from build123d import *

# Parameters (mm, degrees)
ESQUISSE1_R             = 8
ESQUISSE1_R_2           = 1.6
BOSS_EXTRU_1_DEPTH      = 4
ESQUISSE3_R             = 1.6
ENL_V_MAT_EXTRU_1_DEPTH = 10
ENL_V_MAT_EXTRU_2_DEPTH = 5
ESQUISSE5_R             = 1.6
ENL_V_MAT_EXTRU_4_DEPTH = 5
ESQUISSE6_R             = 1.6
ESQUISSE6_R_2           = 1.621897971
ENL_V_MAT_EXTRU_5_DEPTH = 5
ENL_V_MAT_EXTRU_6_DEPTH = 5


with BuildPart() as part:
    # Esquisse1 → Boss.-Extru.1 (new body)
    with BuildSketch(Plane(origin=(0, 0, 0), x_dir=(1, 0, 0), z_dir=(0, 1, 0))):
        Polygon((-150, 0), (-150, 260), (-110, 300), (110, 300), (150, 260), (150, 0), align=None)
        with Locations(Location((-119.984856992, 30, 0), (0, 0, 270))):
            Circle(ESQUISSE1_R, mode=Mode.SUBTRACT)
        with Locations(Location((-120, 268, 0), (0, 0, 270))):
            Circle(ESQUISSE1_R, mode=Mode.SUBTRACT)
        with Locations(Location((120, 269.55960862, 0), (0, 0, 270))):
            Circle(ESQUISSE1_R, mode=Mode.SUBTRACT)
        with Locations(Location((-111.514718626, 276.485281374, 0), (0, 0, 270))):
            Circle(ESQUISSE1_R_2, mode=Mode.SUBTRACT)
        with Locations(Location((-128.485281374, 259.514718626, 0), (0, 0, 270))):
            Circle(ESQUISSE1_R_2, mode=Mode.SUBTRACT)
        with Locations(Location((111.514718626, 278.044889994, 0), (0, 0, 270))):
            Circle(ESQUISSE1_R_2, mode=Mode.SUBTRACT)
        with Locations(Location((128.485281374, 261.074327245, 0), (0, 0, 270))):
            Circle(ESQUISSE1_R_2, mode=Mode.SUBTRACT)
        with Locations(Location((120, 30, 0), (0, 0, 270))):
            Circle(ESQUISSE1_R, mode=Mode.SUBTRACT)
        with Locations(Location((120, 42, 0), (0, 0, 270))):
            Circle(ESQUISSE1_R_2, mode=Mode.SUBTRACT)
        with Locations(Location((-119.984856992, 42, 0), (0, 0, 270))):
            Circle(ESQUISSE1_R_2, mode=Mode.SUBTRACT)
        with Locations(Location((-119.984856992, 18, 0), (0, 0, 270))):
            Circle(ESQUISSE1_R_2, mode=Mode.SUBTRACT)
        with Locations(Location((120, 18, 0), (0, 0, 270))):
            Circle(ESQUISSE1_R_2, mode=Mode.SUBTRACT)
        with Locations(Location((-131.984856992, 30, 0), (0, 0, 270))):
            Circle(ESQUISSE1_R_2, mode=Mode.SUBTRACT)
        with Locations(Location((-107.984856992, 30, 0), (0, 0, 270))):
            Circle(ESQUISSE1_R_2, mode=Mode.SUBTRACT)
        with Locations(Location((108, 30, 0), (0, 0, 270))):
            Circle(ESQUISSE1_R_2, mode=Mode.SUBTRACT)
        with Locations(Location((132, 30, 0), (0, 0, 270))):
            Circle(ESQUISSE1_R_2, mode=Mode.SUBTRACT)
    extrude(amount=BOSS_EXTRU_1_DEPTH)

    # Esquisse3 → Enl_v. mat.-Extru.1 (cut)
    with BuildSketch(Plane(origin=(0, 4, 0), x_dir=(1, 0, 0), z_dir=(0, 1, 0))):
        with Locations(Location((-9, 113, 0), (0, 0, 270))):
            Circle(ESQUISSE3_R)
        with Locations(Location((-6, 179, 0), (0, 0, 270))):
            Circle(ESQUISSE3_R)
        with Locations(Location((-39, 179, 0), (0, 0, 270))):
            Circle(ESQUISSE3_R)
        with Locations(Location((-36, 113, 0), (0, 0, 270))):
            Circle(ESQUISSE3_R)
        with Locations(Location((9, 187, 0), (0, 0, 270))):
            Circle(ESQUISSE3_R)
        with Locations(Location((36, 187, 0), (0, 0, 270))):
            Circle(ESQUISSE3_R)
        with Locations(Location((39, 121, 0), (0, 0, 270))):
            Circle(ESQUISSE3_R)
        with Locations(Location((6, 121, 0), (0, 0, 270))):
            Circle(ESQUISSE3_R)
    enl_v_mat_extru_1 = extrude(amount=-ENL_V_MAT_EXTRU_1_DEPTH, mode=Mode.SUBTRACT)

    # Esquisse4 → Enl_v. mat.-Extru.2 (cut)
    with BuildSketch(Plane(origin=(0, 4, 0), x_dir=(1, 0, 0), z_dir=(0, 1, 0))):
        Polygon((-81, 118), (-45, 118), (-45, 150), (-45, 182), (-81, 182), align=None)
        Polygon((45, 150), (45, 182), (81, 182), (81, 118), (45, 118), align=None)
    extrude(amount=-ENL_V_MAT_EXTRU_2_DEPTH, mode=Mode.SUBTRACT)

    # Sym_trie1: Enl_v. mat.-Extru.1 across plane
    add(enl_v_mat_extru_1.mirror(Plane(origin=(0, 0, 0), x_dir=(0, 0, 1), z_dir=(1, 0, 0))), mode=Mode.SUBTRACT)

    # Esquisse5 → Enl_v. mat.-Extru.4 (cut)
    with BuildSketch(Plane(origin=(0, 4, 0), x_dir=(1, 0, 0), z_dir=(0, 1, 0))):
        with Locations(Location((-42, 224, 0), (0, 0, 270))):
            Circle(ESQUISSE5_R)
        with Locations(Location((-34, 224, 0), (0, 0, 270))):
            Circle(ESQUISSE5_R)
        with Locations(Location((34, 76, 0), (0, 0, 270))):
            Circle(ESQUISSE5_R)
        with Locations(Location((42, 76, 0), (0, 0, 270))):
            Circle(ESQUISSE5_R)
        with Locations(Location((91, 114, 0), (0, 0, 270))):
            Circle(ESQUISSE5_R)
        with Locations(Location((91, 76, 0), (0, 0, 270))):
            Circle(ESQUISSE5_R)
        with Locations(Location((-91, 224, 0), (0, 0, 270))):
            Circle(ESQUISSE5_R)
        with Locations(Location((-91, 186, 0), (0, 0, 270))):
            Circle(ESQUISSE5_R)
    enl_v_mat_extru_4 = extrude(amount=-ENL_V_MAT_EXTRU_4_DEPTH, mode=Mode.SUBTRACT)

    # Sym_trie4: Enl_v. mat.-Extru.4 across plane
    add(enl_v_mat_extru_4.mirror(Plane(origin=(0, 0, 0), x_dir=(0, 0, 1), z_dir=(1, 0, 0))), mode=Mode.SUBTRACT)

    # Esquisse6 → Enl_v. mat.-Extru.5 (cut)
    with BuildSketch(Plane(origin=(0, 4, 0), x_dir=(1, 0, 0), z_dir=(0, 1, 0))):
        with Locations(Location((-102, 112, 0), (0, 0, 270))):
            Circle(ESQUISSE6_R)
        with Locations(Location((-102, 90, 0), (0, 0, 270))):
            Circle(ESQUISSE6_R)
        with Locations(Location((102, 188, 0), (0, 0, 270))):
            Circle(ESQUISSE6_R_2)
        with Locations(Location((102, 210, 0), (0, 0, 270))):
            Circle(ESQUISSE6_R)
        with Locations(Location((-130.5, 112, 0), (0, 0, 270))):
            Circle(ESQUISSE6_R)
        with Locations(Location((-130.5, 90, 0), (0, 0, 270))):
            Circle(ESQUISSE6_R)
        with Locations(Location((130.5, 210, 0), (0, 0, 270))):
            Circle(ESQUISSE6_R)
        with Locations(Location((130.5, 188, 0), (0, 0, 270))):
            Circle(ESQUISSE6_R)
    enl_v_mat_extru_5 = extrude(amount=-ENL_V_MAT_EXTRU_5_DEPTH, mode=Mode.SUBTRACT)

    # Esquisse7 → Enl_v. mat.-Extru.6 (cut)
    with BuildSketch(Plane(origin=(0, 4, 0), x_dir=(1, 0, 0), z_dir=(0, 1, 0))):
        Polygon((-122, 150), (-122, 182), (-132, 182), (-132, 118), (-122, 118), align=None)
    enl_v_mat_extru_6 = extrude(amount=-ENL_V_MAT_EXTRU_6_DEPTH, mode=Mode.SUBTRACT)

    # Sym_trie5: Enl_v. mat.-Extru.6 across plane
    add(enl_v_mat_extru_6.mirror(Plane(origin=(0, 0, 0), x_dir=(0, 0, 1), z_dir=(1, 0, 0))), mode=Mode.SUBTRACT)

    # Sym_trie6: Enl_v. mat.-Extru.5 across plane
    add(enl_v_mat_extru_5.mirror(Plane(origin=(0, 0, 0), x_dir=(0, 0, 1), z_dir=(1, 0, 0))), mode=Mode.SUBTRACT)


solid = part.part
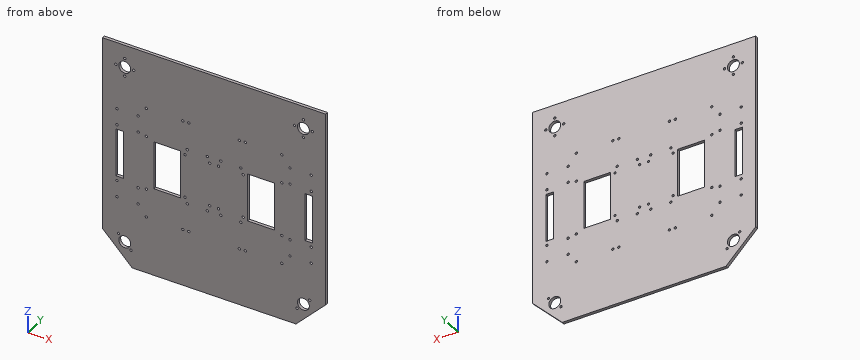
Input: part model. Units: mm. Frame: model coordinates. Coordinates: 2 decimals unless noted, no trailing zeros. Write each loop counter-clockwise with the first axis right and the second up, starting at its lowest first coordinate (ties: lowest second). Pieces come first, ordered by that corner, then holes. Notation, with made-up numbers: M 20,-15.75 L 52,-15.75 A7 cw 52,-7.75 Z; hole C -22.75,0 d6. An arc over 180 degrees is marked long. Answer as a JSON object with one key per item and string values. Group by question number.
(1) Section C-C on y = 2.6. Give the number of separate pieces and of enclosed holes in the cut face, plus the area to 3 significant figures.
(2) Contact query for a flat-ended pin moving along its axis: P1, Ø5, axis at x = -6, z = -179, coming from the -Y side. Output: stop coordinate, or through.
(3) Section B-B on x = 73.5. Output: boundary loops of the cut face in (y, z), plus the area to 3 significant figures.
(4) Ray query, line 1 along Z through (x, y) = (-91, 1); line 2 along X through (y, z) = (2.45, -161.5); line 3 along X through (y, z) = (2.95, -90). Return the intervals inside material, ascending. Write a range as [from, to].
(5) Section A-A on z = -166.5. Output: boundary loops of the cut face in (x, y).
Result set:
{
 "1": {"separate pieces": "1", "enclosed holes": "68", "area": "81,200 mm2"},
 "2": {"P1": "stops at y = 0"},
 "3": {"outline": "M 0,-300 L 4,-300 L 4,-182 L 0,-182 Z; M 0,-118 L 4,-118 L 4,0 L 0,0 Z", "area": "944 mm2"},
 "4": {"line 1": "z = [-300, -225.6], [-222.4, -187.6], [-184.4, -115.6], [-112.4, -77.6], [-74.4, 0]", "line 2": "x = [-150, -132], [-122, -81], [-45, 45], [81, 122], [132, 150]", "line 3": "x = [-150, -132.1], [-128.9, -103.6], [-100.4, 100.4], [103.6, 128.9], [132.1, 150]"},
 "5": {"outline": "M -150,0 L -132,0 L -132,4 L -150,4 Z; M -122,0 L -81,0 L -81,4 L -122,4 Z; M -45,0 L 45,0 L 45,4 L -45,4 Z; M 81,0 L 122,0 L 122,4 L 81,4 Z; M 132,0 L 150,0 L 150,4 L 132,4 Z"}
}
